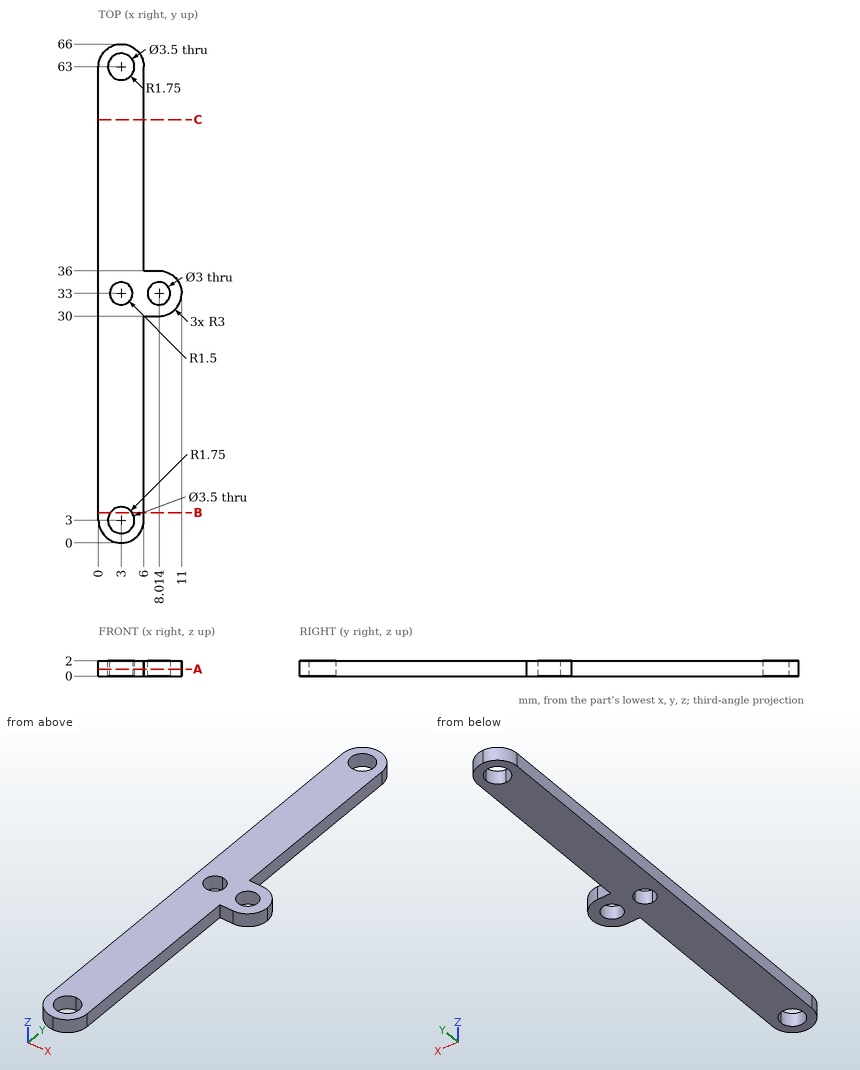
Print and shaded views of the part. All mm, measured from the part's lowest x, y and z. Give positions to 0.01 mm unless a question says otherwise; leave off trailing zeros. Write each loop counter-clockwise with the first axis right and the second up, starting at its lowest first coordinate (ties: lowest second). Pieces come first, ordered by that corner, then holes. Notation, with made-up numbers: (24.5, -18.75) -> (81.5, -18.75) arc R15 cw to (81.5, 10.25) -> close; hole circle Ø4 at (71, 66). An arc over 180 degrees is marked (long way). Use CSV: the item, a comma, the result in double quotes. Start each with the question number.
1) Cut at C-C on y = 56. List the corners of the cut face in (x, z).
2) Cut at A-A on z = 0.9. Count the separate pieces of the cut face and the enclosed holes in it, plus the area to 3 significant figures.
3) Pin check, flat tips, straight feed: P1, Ø0.6, axis at y = 19.5, z = 1.5, coming from the +X side; P2, Ø4, axis at x = 9, y = 37.5, coming from the +Z side; P3, Ø0.6, axis at x = 7, z = 1, coming from the -Y side; P4, Ø3, axis at x = 3, y = 63, coming from the -Z side. Stop position of each tip, or through.
4) Cut at B-B on y = 4. List the corners of the cut face in (x, z).
5) Drill centre lines: L1, parallel to X at y = 3, z = 1.2; L2, parallel to X at y = 32, z = 0.9; L3, parallel to Y at x = 3.5, z = 0.2. Where is each one in solid material? Low to high.
Final values:
1,outline,"(0, 0) -> (6, 0) -> (6, 2) -> (0, 2) -> close"
2,separate pieces,"1"
2,enclosed holes,"4"
2,area,"381 mm2"
3,P1,"stops at x = 6"
3,P2,"stops at z = 2"
3,P3,"stops at y = 30"
3,P4,"passes through"
4,outline,"(0, 0) -> (1.56, 0) -> (1.56, 2) -> (0, 2) -> close; (4.44, 0) -> (6, 0) -> (6, 2) -> (4.44, 2) -> close"
5,L1,"x = 0 to 1.25, 4.75 to 6"
5,L2,"x = 0 to 1.88, 4.12 to 6.9, 9.13 to 10.83"
5,L3,"y = 0.04 to 1.32, 4.68 to 31.59, 34.41 to 61.32, 64.68 to 65.96"
